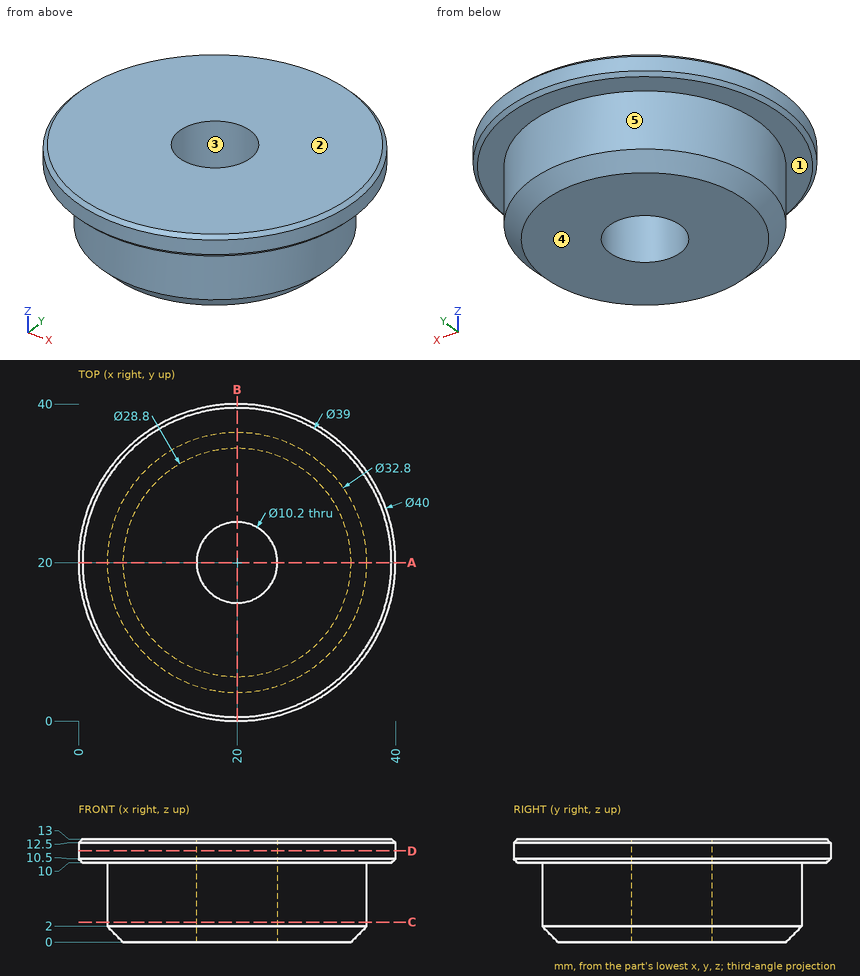
Study the drawing (mm; zero at the part's minimum x, y, z) and answer. A direction names the side the tool comes from. Coordinates: 2 decimals unless noted, no trailing zeros. Write each loop counter-clockwise with the first axis right and the second up, starting at its lowest first coordinate (ties: lowest second). Pieces come first, ordered by that corner, then holes. Notation, with made-up numbers: (-24, -3) - (25, -3) arc R8 ccw to (25, 5) - close; hole circle Ø2 at (-10, -27.5). An arc over 180 degrees is marked (long way). Return JSON: item names as keys, results as strings. Group by question number.
1. Straight lines are drawn through the part: L1, parallel to Y at x = 20, z = 6; L2, parallel to Y at x = 20, z = 10.5; L3, parallel to Z at x = 11.5, y = 35. For each, find the intervals that lie inside material, in ascending order.
2. A cutting plane is placed at C-C, the plane z = 2.5. Determine the outline of the cut face in (x, y).
3. Which of the six approach directions +Z, -Z, +X, -X, +Y, -Y give full straight-line access (tool end or side, diameter ignored) to the marked faces 1 and 2?
4. Given pin 1 (5 mm diameter, centred on x = 26, z = 4, fed in from -Y); pin 2 (1.5 mm diameter, centred on y = 35, z = 5, fed in from -X); pin 3 (12 mm diameter, centred on x = 24.5, y = 9, fed in from -Z); pin 4 (2 mm diameter, centred on x = 9, z = 7, fed in from +Y), each flat-ended and moving along its own axis, determine where each tip first touches the part or whether it passes through.
5. A cutting plane is placed at A-A, the plane y = 20. Determine the outline of the cut face in (x, z), plus the area to 3 significant figures.
6. Determine the mould class of the marked faces 3, 4 and 5 for opening direction Y: released by +Y, released by -Y, zero draft, split by the parting line, or undercut.
7. A cutting plane is placed at D-D, the plane z = 11.5. Determine the outline of the cut face in (x, y), plus the area to 3 significant figures.
Ans:
{
 "1": {"L1": "3.6 to 14.9, 25.1 to 36.4", "L2": "0 to 14.9, 25.1 to 40", "L3": "10 to 13"},
 "2": {"outline": "circle Ø32.8 at (20, 20); hole circle Ø10.2 at (20, 20)"},
 "3": {"face 1": "-Z", "face 2": "+Z, +X, -X, +Y, -Y"},
 "4": {"pin 1": "y = 3.98", "pin 2": "x = 11.88", "pin 3": "z = 0", "pin 4": "y = 33"},
 "5": {"outline": "(0, 10.5) - (0.5, 10) - (3.6, 10) - (3.6, 2) - (5.6, 0) - (14.9, 0) - (14.9, 13) - (0.5, 13) - (0, 12.5) - close; (25.1, 0) - (34.4, 0) - (36.4, 2) - (36.4, 10) - (39.5, 10) - (40, 10.5) - (40, 12.5) - (39.5, 13) - (25.1, 13) - close", "area": "311 mm²"},
 "6": {"face 3": "undercut", "face 4": "zero draft", "face 5": "split by the parting line"},
 "7": {"outline": "circle Ø40 at (20, 20); hole circle Ø10.2 at (20, 20)", "area": "1,170 mm²"}
}
